The model under review builds one solid part; all positions refer to its coordinate system, in mm. A direction names the side the tool comes from. Coordinates: 2 decimals unless noted, no trailing zeros. Loops run counter-clockwise (first coordinate to the right, second up) from the corner with the lowest first, then second, coordinate; pieces in that order, holes last. Notation, with made-up numbers: M -34.75,42 L -23.75,42 A29 ccw -23.75,76 Z; hole C 40,30 d7. An arc over 180 degrees is marked long. Write item = value, one per line. Start each with the question number.
Q1. We need section C-C on y = 11.5. Give the boundary of the cut face in (x, z), and give its area (3 significant figures).
Q2. For faces 5 (the face through (7, 1.5, -16)), 6 (the face through (26, 1, -11)), list the 3-axis set-ups (+Z, -Z, +X, -X, +Y, -Y) from which the entire face can be reached by the end or side of a thin tool; tool diameter is ignored.
Q3. We need section A-A on z = -15.75. Give the boundary of the cut face in (x, y).
Q4. Mouldability with a two-part tool opening along X and no side actions: class faces 1 (the face through (4.708, 16.586, 0.74)), 2 (the face through (25.57, 0.76, -31.05)), 3 (the face through (16, 12, 0)), 4 (the face through (22.983, 0.74, -22.49)) as released by +X, released by -X, zero draft, split by the parting line, or undercut.
Q5. Clearance check with flat-ended pins moving along their axes: pin 1 Ø6 at (x, y) = (9, 24.5) entering from -Z; pin 2 Ø4 at (x, z) = (14.5, -12.5) entering from +Y. State where each tip first meets the part, or that it passes through.
Q6. We need section B-B on x = 13. Give the boundary of the cut face in (y, z).
Q7. Wall thickness on probe 1 along X at (y, z) = (1.05, -8.75); probe 2 along Y at (x, z) = (13, 0.9); probe 3 along Z at (x, y) = (8, 13.25): over which ranges is each line inside the solid? List them lowest first.
Q8. We need section D-D on z = -8.75. Give the boundary of the cut face in (x, y).
from build123d import *

# Parameters (mm, degrees)
BOSS_EXTRUDE1_DEPTH = 1.5
SKETCH2_R           = 1.6
SKETCH2_R_2         = 4
CUT_EXTRUDE1_DEPTH  = 39.23937761
SKETCH3_W           = 26
SKETCH3_H           = 1.5
BOSS_EXTRUDE4_DEPTH = 31.5
SKETCH4_R           = 5
SKETCH4_R_2         = 2
CUT_EXTRUDE2_DEPTH  = 50.520197899
FILLET1_R           = 1.5


with BuildPart() as part:
    # Sketch1 → Boss-Extrude1 (new body)
    with BuildSketch(Plane.XY):
        with BuildLine():
            Line((0, 0), (26, 0))
            Line((26, 0), (26, 15))
            ThreePointArc((26, 15), (13, 28), (0, 15))
            Line((0, 15), (0, 0))
        make_face()
    extrude(amount=BOSS_EXTRUDE1_DEPTH)

    # Sketch2 → Cut-Extrude1 (cut, through all)
    with BuildSketch(Plane(origin=(0, 0, 0), x_dir=(-1, 0, 0), z_dir=(0, 0, -1))):
        with Locations((-21.5, 15)):
            Circle(SKETCH2_R)
        with Locations((-13, 15)):
            Circle(SKETCH2_R_2)
        with Locations((-4.5, 15)):
            Circle(SKETCH2_R)
    extrude(amount=-CUT_EXTRUDE1_DEPTH, mode=Mode.SUBTRACT)

    # Sketch3 → Boss-Extrude4 (add)
    with BuildSketch(Plane(origin=(0, 0, 0), x_dir=(-1, 0, 0), z_dir=(0, 0, -1))):
        with Locations((-13, 0.75)):
            Rectangle(SKETCH3_W, SKETCH3_H)
    extrude(amount=BOSS_EXTRUDE4_DEPTH)

    # Sketch4 → Cut-Extrude2 (cut, through all)
    with BuildSketch(Plane.XZ):
        with Locations(Location((13, -15.75, 0), (0, 0, 270))):
            Circle(SKETCH4_R)
        with Locations(Location((5, -8.75, 0), (0, 0, 270))):
            Circle(SKETCH4_R_2)
        with Locations(Location((21, -8.75, 0), (0, 0, 270))):
            Circle(SKETCH4_R_2)
        with Locations(Location((21, -22.75, 0), (0, 0, 270))):
            Circle(SKETCH4_R_2)
        with Locations(Location((5, -22.75, 0), (0, 0, 270))):
            Circle(SKETCH4_R_2)
    extrude(amount=-CUT_EXTRUDE2_DEPTH, mode=Mode.SUBTRACT)

    # Fillet1
    fillet1_edges = [part.edges().sort_by_distance(p)[0] for p in [
        (26, 0.75, -31.5),
        (0, 0.75, -31.5),
    ]]
    fillet(fillet1_edges, radius=FILLET1_R)


solid = part.part
Returned:
q1.outline = M 0,0 L 11.06,0 L 11.06,1.5 L 0,1.5 Z; M 14.94,0 L 26,0 L 26,1.5 L 14.94,1.5 Z
q1.area = 33.2 mm^2
q2.face_5 = -Z, +X, -X, +Y
q2.face_6 = +Z, -Z, +X, +Y, -Y
q3.outline = M 0,0 L 8,0 L 8,1.5 L 0,1.5 Z; M 18,0 L 26,0 L 26,1.5 L 18,1.5 Z
q4.face_1 = undercut
q4.face_2 = released by +X
q4.face_3 = zero draft
q4.face_4 = undercut
q5.pin_1 = 0
q5.pin_2 = 1.5
q6.outline = M 0,-31.5 L 1.5,-31.5 L 1.5,-20.75 L 0,-20.75 Z; M 0,-10.75 L 1.5,-10.75 L 1.5,0 L 11,0 L 11,1.5 L 0,1.5 Z; M 19,0 L 28,0 L 28,1.5 L 19,1.5 Z
q7.probe_1 = 0 to 3, 7 to 19, 23 to 26
q7.probe_2 = 0 to 11, 19 to 28
q7.probe_3 = 0 to 1.5
q8.outline = M 0,0 L 3,0 L 3,1.5 L 0,1.5 Z; M 7,0 L 19,0 L 19,1.5 L 7,1.5 Z; M 23,0 L 26,0 L 26,1.5 L 23,1.5 Z
